```python
from build123d import *

# Parameters (mm, degrees)
SKETCH1_W           = 40
SKETCH1_H           = 10
BOSS_EXTRUDE1_DEPTH = 40
FILLET1_R           = 15
SKETCH3_R           = 2
CUT_EXTRUDE1_DEPTH  = 10
SKETCH7_W           = 15
SKETCH7_H           = 60
BOSS_EXTRUDE5_DEPTH = 8
SKETCH8_R           = 2.5
BOSS_EXTRUDE6_DEPTH = 4
SKETCH9_R           = 1
BOSS_EXTRUDE7_DEPTH = 8
FILLET3_R           = 5


with BuildPart() as part:
    # Sketch1 → Boss-Extrude1 (new body)
    with BuildSketch(Plane(origin=(0, 0, 0), x_dir=(1, 0, 0), z_dir=(0, 1, 0))):
        Rectangle(SKETCH1_W, SKETCH1_H)
    extrude(amount=BOSS_EXTRUDE1_DEPTH)

    # Fillet1
    fillet1_edges = [part.edges().sort_by_distance(p)[0] for p in [
        (-20, 40, 0),
        (20, 40, 0),
    ]]
    fillet(fillet1_edges, radius=FILLET1_R)

    # Sketch3 → Cut-Extrude1 (cut)
    with BuildSketch(Plane.XY.offset(5)):
        with Locations((15, 10)):
            Circle(SKETCH3_R)
        with Locations((-15, 10)):
            Circle(SKETCH3_R)
    extrude(amount=-CUT_EXTRUDE1_DEPTH, mode=Mode.SUBTRACT)

    # Sketch7 → Boss-Extrude5 (add)
    with BuildSketch(Plane.XY.offset(5)):
        Rectangle(SKETCH7_W, SKETCH7_H)
    extrude(amount=BOSS_EXTRUDE5_DEPTH)

    # Sketch8 → Boss-Extrude6 (add)
    with BuildSketch(Plane.XZ.offset(30)):
        with Locations((0, 9)):
            Circle(SKETCH8_R)
    extrude(amount=BOSS_EXTRUDE6_DEPTH)

    # Sketch9 → Boss-Extrude7 (add)
    with BuildSketch(Plane.XZ.offset(34)):
        with Locations((0, 9)):
            Circle(SKETCH9_R)
    extrude(amount=BOSS_EXTRUDE7_DEPTH)

    # Fillet3
    fillet3_edges = [part.edges().sort_by_distance(p)[0] for p in [
        (7.5, 0, 13),
        (-7.5, 0, 13),
    ]]
    fillet(fillet3_edges, radius=FILLET3_R)


solid = part.part
```
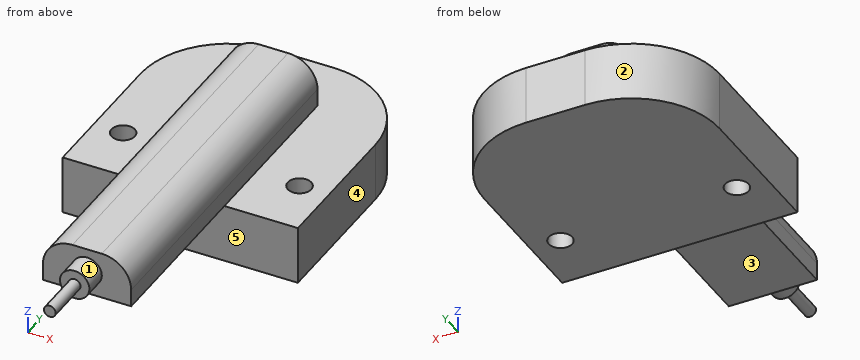
Can you work these out from the model? Positions are in its coordinate system, mm. Face numbers are marked on the shaded views. A direction names the side the tool comes from. Coordinates: 2 decimals unless noted, no trailing zeros. Loops run counter-clockwise (first coordinate to the right, second up) from the corner with the lowest first, then second, coordinate; pieces in that order, holes last. Notation, with made-up numbers: (59, -12.75) -> (94, -12.75) arc R16 cw to (94, 8.25) -> close; hole circle Ø3 at (78, 66). An arc over 180 degrees is marked (long way). Answer as a JSON object with one key per item and string values.
1) If I drill on line 1 (Y direction, x = -4, z = 5.5); line 2 (Z direction, x = -17.5, y = 1.5); line 3 (Y direction, x = -15, z = -2), over which ranges is the centre line in solid material (lowest first)?
Results:
{"line 1": "y = -30 to 30", "line 2": "z = -5 to 5", "line 3": "y = 0 to 8, 12 to 36.18"}
2) Imagine slicing it at C-C (z = -1.75). Please give me the cut outline in (x, y).
Results:
{"outline": "(-20, 0) -> (20, 0) -> (20, 25) arc R15 ccw to (5, 40) -> (-5, 40) arc R15 ccw to (-20, 25) -> close; hole circle Ø4 at (-15, 10); hole circle Ø4 at (15, 10)"}
3) For the marked faces 4 and 5, which set-ups out of +Z, -Z, +X, -X, +Y, -Y let a thin tool reach every point of the face, with its end or its side?
Results:
{"face 4": "+Z, -Z, +X, +Y, -Y", "face 5": "-Z, +X, -X, -Y"}
4) Imagine slicing it at A-A (x = 0). Please give me the cut outline in (y, z), then the cut area to 3 significant figures.
Results:
{"outline": "(-42, 8) -> (-34, 8) -> (-34, 6.5) -> (-30, 6.5) -> (-30, 5) -> (0, 5) -> (0, -5) -> (40, -5) -> (40, 5) -> (30, 5) -> (30, 13) -> (-30, 13) -> (-30, 11.5) -> (-34, 11.5) -> (-34, 10) -> (-42, 10) -> close", "area": "916 mm^2"}
5) Imagine slicing it at D-D (y = 11). Please give me the cut outline in (x, z), then the cut area to 3 significant figures.
Results:
{"outline": "(-20, -5) -> (-16.73, -5) -> (-16.73, 5) -> (-20, 5) -> close; (-13.27, -5) -> (13.27, -5) -> (13.27, 5) -> (7.5, 5) -> (7.5, 8) arc R5 ccw to (2.5, 13) -> (-2.5, 13) arc R5 ccw to (-7.5, 8) -> (-7.5, 5) -> (-13.27, 5) -> close; (16.73, -5) -> (20, -5) -> (20, 5) -> (16.73, 5) -> close", "area": "440 mm^2"}
6) Imagine slicing it at B-B (x = 15). Please give me the cut outline in (y, z).
Results:
{"outline": "(0, -5) -> (8, -5) -> (8, 5) -> (0, 5) -> close; (12, -5) -> (36.18, -5) -> (36.18, 5) -> (12, 5) -> close"}
7) Thinking about a two-plate mould opening in X: for the marked faces 1, 2 and 3, which applies, pulls with the +X half, pulls with the -X half, needs draft (parallel to the pull), parting line crosses it, or undercut?
Results:
{"face 1": "parting line crosses it", "face 2": "pulls with the -X half", "face 3": "needs draft"}
8) For P1, Ø12, axis at x = 8, y = -10.5, coming from the +Z side; P2, Ø16.5, axis at x = -3, y = -20.5, coming from the -Z side; P3, Ø1.5, axis at y = -8, z = 4.5, coming from the +X side; P4, Ø6, axis at x = 8, y = -17.5, coming from the +Z side, each with a flat end and sliding along its axis, tell me the tip position at first contact or that it passes through.
Results:
{"P1": "stops at z = 13", "P2": "stops at z = 5", "P3": "stops at x = 7.5", "P4": "stops at z = 12.33"}
